Work out the finished part from the listing and answer in its coordinate system (mm). Coordinates: 2 decimals unless noted, no trailing zeros. Write each loop counter-clockwise with the first axis right and the second up, starting at its lowest first coordinate (ties: lowest second). Pieces come first, ordered by that corner, then holes. Notation, with made-up numbers: M 84.5,19 L 138.5,19 A37 ccw 138.5,56 Z; hole C -28,80 d11. An arc over 180 degrees is marked long. Use CSV: the item, a comma, the result in double quotes.
from build123d import *

# Parameters (mm, degrees)
SKETCH1_R           = 45
SKETCH1_R_2         = 4
SKETCH1_R_3         = 0.75
SKETCH1_W           = 5
SKETCH1_H           = 13
BOSS_EXTRUDE1_DEPTH = 5


with BuildPart() as part:
    # Sketch1 → Boss-Extrude1 (new body)
    with BuildSketch(Plane(origin=(0, 0, 0), x_dir=(1, 0, 0), z_dir=(0, 1, 0))):
        Circle(SKETCH1_R)
        Circle(SKETCH1_R_2, mode=Mode.SUBTRACT)
        with Locations((6.368925704, 0.593189593)):
            Circle(SKETCH1_R_3, mode=Mode.SUBTRACT)
        with Locations((0.593189593, -6.368925704)):
            Circle(SKETCH1_R_3, mode=Mode.SUBTRACT)
        with Locations((-0.593189593, 6.368925704)):
            Circle(SKETCH1_R_3, mode=Mode.SUBTRACT)
        with Locations((-6.368925704, -0.593189593)):
            Circle(SKETCH1_R_3, mode=Mode.SUBTRACT)
        with Locations((26.5, -16.682134432)):
            Rectangle(SKETCH1_W, SKETCH1_H, mode=Mode.SUBTRACT)
        with Locations((26.5, 16.682134432)):
            Rectangle(SKETCH1_W, SKETCH1_H, mode=Mode.SUBTRACT)
        with Locations((-26.5, -16.682134432)):
            Rectangle(SKETCH1_W, SKETCH1_H, mode=Mode.SUBTRACT)
        with Locations((26.5, 0)):
            Rectangle(SKETCH1_W, SKETCH1_H, mode=Mode.SUBTRACT)
        with Locations((-26.5, 0)):
            Rectangle(SKETCH1_W, SKETCH1_H, mode=Mode.SUBTRACT)
        with Locations((-26.5, 16.682134432)):
            Rectangle(SKETCH1_W, SKETCH1_H, mode=Mode.SUBTRACT)
    extrude(amount=BOSS_EXTRUDE1_DEPTH)


solid = part.part
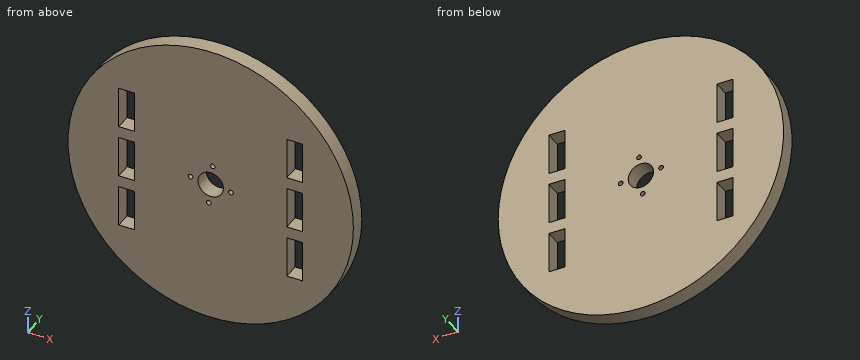
Item 1: The part is cut by section A-A (z = 14). Write down the section's boundary in (x, y), then the cut area to 3 significant figures.
Answer:
outline,"M -42.77,0 L -29,0 L -29,5 L -42.77,5 Z; M -24,0 L 24,0 L 24,5 L -24,5 Z; M 29,0 L 42.77,0 L 42.77,5 L 29,5 Z"
area,"378 mm2"
Item 2: Given pin 1 (2.5 mm diameter, centred on y = 2.5, z = -1.5, fed in from -X); pin 2 (2 mm diameter, centred on y = 2.5, z = 20, fed in from +X); pin 3 (1.5 mm diameter, centred on x = 27, y = 1.5, fed in from +Z), each flat-ended and moving along its own axis, determine where each tip first touches the part or whether it passes through.
Answer:
pin 1,"stops at x = -45"
pin 2,"stops at x = 40.79"
pin 3,"stops at z = 36.55"
Item 3: The part is cut by section D-D (z = -17). Write down the section's boundary in (x, y), then the cut area to 3 significant figures.
Answer:
outline,"M -41.67,0 L -29,0 L -29,5 L -41.67,5 Z; M -24,0 L 24,0 L 24,5 L -24,5 Z; M 29,0 L 41.67,0 L 41.67,5 L 29,5 Z"
area,"367 mm2"
Item 4: Consider probe 1 along Z at (x, y) = (0, 2); probe 2 along X at (y, z) = (0.85, 13.5); probe 3 along X at (y, z) = (2.5, 5). Determine where each line is inside the solid, lowest interval first.
Answer:
probe 1,"z = -45 to -6.83, -5.91 to -4, 4 to 5.91, 6.83 to 45"
probe 2,"x = -42.93 to -29, -24 to 24, 29 to 42.93"
probe 3,"x = -44.72 to -29, -24 to 24, 29 to 44.72"
Item 5: The part is cut by section C-C (x = -25.5). Write down the section's boundary in (y, z), then the cut area to 3 significant figures.
Answer:
outline,"M 0,-37.08 L 5,-37.08 L 5,-23.18 L 0,-23.18 Z; M 0,-10.18 L 5,-10.18 L 5,-6.5 L 0,-6.5 Z; M 0,6.5 L 5,6.5 L 5,10.18 L 0,10.18 Z; M 0,23.18 L 5,23.18 L 5,37.08 L 0,37.08 Z"
area,"176 mm2"
Item 6: The part is cut by section B-B (y = 1.9). Count the separate pieces of the cut face and the enclosed holes in it, then the cut area to 3 significant figures.
Answer:
separate pieces,"1"
enclosed holes,"11"
area,"5,910 mm2"
